```python
from build123d import *

# Parameters (mm, degrees)
F1_DEPTH      = 50.8
F1_DEPTH_BACK = 25.4
F2_DEPTH      = 25.4


with BuildPart() as f1:
    # F0 (on Front) → F1 (new body, two sides)
    with BuildSketch(Plane.XZ) as f1_sk:
        Polygon((-56.026979, 25.396531), (-56.026979, 50.796531), (-81.007203, 50.796531), (-81.007203, 0), (71.392797, 0), (70.973021, 25.396531), align=None)
    extrude(amount=F1_DEPTH)
    extrude(f1_sk.sketch, amount=-F1_DEPTH_BACK)

    # F0 (on Front) → F2 (join)
    with BuildSketch(Plane.XZ):
        Polygon((70.973021, 25.396531), (-56.026979, 50.796531), (-56.026979, 25.396531), align=None)
    extrude(amount=F2_DEPTH)


solid = f1.part
```
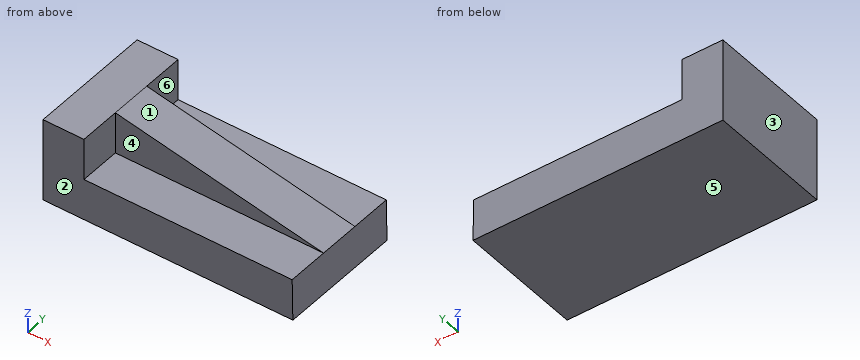
Check sheet for the modelled part. Datum: model origin and axes. Units: mm. Face numbers are marked on the shaded views. A direction names the side the tool comes from. Round coordinates to 2 decimals unless told otherwise and drop trailing zeros. Order: outer loops, then holes, each group sorted by start corner. A loop starts at its lowest first (then second) coordinate and runs counter-clockwise, first axis right, second up. Notation, with made-up numbers: M -3,49 L 15,49 A24 ccw 15,72 Z; hole C 20.25,74.5 d5. An arc over 180 degrees is marked long. Answer in a Markdown table with one row per item.
(1) Section check A-A on y = -42.5. Record the boundary of the cut face in (x, z).
Findings:
| item | result |
|---|---|
| outline | M -81.01,0 L 71.39,0 L 70.97,25.4 L -56.03,25.4 L -56.03,50.8 L -81.01,50.8 Z |
(2) Section check B-B on x = 31.5. Record the boundary of the cut face in (y, z).
Findings:
| item | result |
|---|---|
| outline | M -50.8,0 L 25.4,0 L 25.4,25.4 L 0,25.4 L 0,33.29 L -25.4,33.29 L -25.4,25.4 L -50.8,25.4 Z |
(3) Set-up check for the marked faces 4, 5 and 6: record each of +Z, -Z, +X, -X, +Y, -Y from which the full face is reachable in a straight line by a thin tool's end or side.
Findings:
| item | result |
|---|---|
| face 4 | +Z, +X, -Y |
| face 5 | -Z, +X, -X, +Y, -Y |
| face 6 | +Z, +X, +Y |
(4) Material ranges on line 1 along Z through (x, y) = (49.5, 3); line 2 along Y through (x, z) = (-27.5, 45); line 3 along X through (y, z) = (-30, 47), recorded low to high. Write a range as from..to.
Findings:
| item | result |
|---|---|
| line 1 | z = 0..25.4 |
| line 2 | y = -25.4..0 |
| line 3 | x = -81.01..-56.03 |
(5) Draft check along X on the marked faces 1, 2 and 3. Enter one of: +X half, -X half, draft (parallel to the pull), parting line (faces both ways), or undercut.
Findings:
| item | result |
|---|---|
| face 1 | +X half |
| face 2 | draft |
| face 3 | -X half |
(6) Gauge pin test, flat ends, axial feed: pin 1 (7.5 mm diameter, centred on x = 10, y = 17.5, fed in from +Z); pin 2 (8 mm diameter, centred on y = -32.5, z = 36, fed in from +X); pin 3 (2 mm diameter, centred on x = -21.5, z = 35, fed in from -Y). Record the tip position at first contact, or that the pin passes through.
Findings:
| item | result |
|---|---|
| pin 1 | stops at z = 25.4 |
| pin 2 | stops at x = -56.03 |
| pin 3 | stops at y = -25.4 |
(7) Section check D-D on y = -17. Record the boundary of the cut face in (x, z).
Findings:
| item | result |
|---|---|
| outline | M -81.01,0 L 71.39,0 L 70.97,25.4 L -56.03,50.8 L -81.01,50.8 Z |
(8) Section check C-C on z = 29.5. Record the boundary of the cut face in (x, y), plus the area to 3 significant figures.
Findings:
| item | result |
|---|---|
| outline | M -81.01,-50.8 L -56.03,-50.8 L -56.03,-25.4 L 50.46,-25.4 L 50.46,0 L -56.03,0 L -56.03,25.4 L -81.01,25.4 Z |
| area | 4,610 mm^2 |
